```python
from build123d import *

# Parameters (mm, degrees)
F1_DEPTH = 10
F0_R     = 9.5
F2_DEPTH = 20
F3_DEPTH = 5
F4_R     = 6


with BuildPart() as f1:
    # F0 (on Top) → F1 (new body)
    with BuildSketch(Plane.XY):
        with BuildLine():
            Line((-9, 60), (-9, 42.0475920833))
            ThreePointArc((-9, 42.0475920833), (-6.5112727326, 42.5041565897), (-4, 42.8135492572))
            Line((-4, 42.8135492572), (-4, 60))
            ThreePointArc((-4, 60), (0, 64), (4, 60))
            Line((4, 60), (4, 42.8135492572))
            ThreePointArc((4, 42.8135492572), (6.5112727326, 42.5041565897), (9, 42.0475920833))
            Line((9, 42.0475920833), (9, 60))
            ThreePointArc((9, 60), (0, 69), (-9, 60))
        make_face()
        with BuildLine():
            Line((-9, 42.0475920833), (-9, 14.4222051019))
            ThreePointArc((-9, 14.4222051019), (0, 17), (9, 14.4222051019))
            Line((9, 14.4222051019), (9, 42.0475920833))
            ThreePointArc((9, 42.0475920833), (6.5112727326, 42.5041565897), (4, 42.8135492572))
            Line((4, 42.8135492572), (4, 33))
            ThreePointArc((4, 33), (0, 29), (-4, 33))
            Line((-4, 33), (-4, 42.8135492572))
            ThreePointArc((-4, 42.8135492572), (-6.5112727326, 42.5041565897), (-9, 42.0475920833))
        make_face()
    extrude(amount=F1_DEPTH)

    # F0 (on Top) → F2 (join)
    with BuildSketch(Plane.XY):
        with BuildLine():
            ThreePointArc((-9, 14.4222051019), (-8.2462112512, -14.8660687473), (17, 0))
            ThreePointArc((17, 0), (16.9906697283, 0.5631537833), (16.9626891549, 1.1256894045))
            ThreePointArc((16.9626891549, 1.1256894045), (14.5847399518, 8.7341491022), (9, 14.4222051019))
            ThreePointArc((9, 14.4222051019), (0, 17), (-9, 14.4222051019))
        make_face()
        Circle(F0_R, mode=Mode.SUBTRACT)
    extrude(amount=F2_DEPTH)

    # F0 (on Top) → F3 (join)
    with BuildSketch(Plane.XY):
        with BuildLine():
            ThreePointArc((9, 14.4222051019), (14.5847399518, 8.7341491022), (16.9626891549, 1.1256894045))
            ThreePointArc((16.9626891549, 1.1256894045), (19.3722847508, 6.3399805993), (25.0605147601, 7.1393697171))
            ThreePointArc((25.0605147601, 7.1393697171), (36.2055537239, 10.0321400586), (37.2390923627, 21.5))
            ThreePointArc((37.2390923627, 21.5), (25.2994921043, 34.7697526489), (9, 42.0475920833))
            Line((9, 42.0475920833), (9, 14.4222051019))
        make_face()
        with BuildLine():
            ThreePointArc((32.04293994, 18.5), (30.5788383249, 13.0358983849), (25.1147367097, 14.5))
            ThreePointArc((25.1147367097, 14.5), (20.5060966544, 20.5060966544), (14.5, 25.1147367097))
            ThreePointArc((14.5, 25.1147367097), (13.0358983849, 30.5788383249), (18.5, 32.04293994))
            ThreePointArc((18.5, 32.04293994), (26.1629509039, 26.1629509039), (32.04293994, 18.5))
        make_face(mode=Mode.SUBTRACT)
    extrude(amount=F3_DEPTH)

    # F4
    f4_edges = [f1.edges().sort_by_distance(p)[0] for p in [
        (9, 42.047592, 2.5),
    ]]
    fillet(f4_edges, radius=F4_R)


solid = f1.part
```
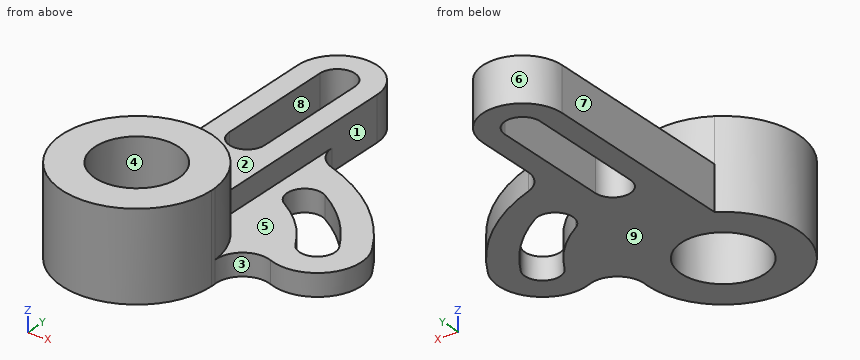
Check sheet for the modelled part. Datum: model origin and axes. Units: mm. Face numbers are marked on the shaded views. A direction names the side the tool comes from. Round coordinates to 2 decimals unless told otherwise and drop trailing zeros. Loops run counter-clockwise (first coordinate to the right, second up) from the corner with the lowest first, then second, coordinate; pieces in that order, holes last. Notation, with made-up numbers: (-31, 48.25) -> (-5, 48.25) arc R24 cw to (-5, 72.25) -> close; hole circle Ø11 at (-5.5, -12). An arc over 180 degrees is marked (long way). Answer in a Markdown table with one row per item.
Q1. Sectioned sample at A-A on y = 54. Enter the section's corners in (x, z).
Data:
| item | result |
|---|---|
| outline | (-9, 0) -> (-4, 0) -> (-4, 10) -> (-9, 10) -> close; (4, 0) -> (9, 0) -> (9, 10) -> (4, 10) -> close |
Q2. Go/stop test with flat-tipped pins: P1, Ø5, axis at y = 52.5, z = 5.5, coming from the -X side; P2, Ø14.5, axis at x = -1, y = 53, coming from the +Z side; P3, Ø11, axis at y = 36.5, z = 5, coming from the +X side; P4, Ø8, axis at y = 44, z = 16, coming from the -X side. Record where each tip stops, or that it passes through.
Data:
| item | result |
|---|---|
| P1 | stops at x = -9 |
| P2 | stops at z = 10 |
| P3 | stops at x = 29.8 |
| P4 | passes through |
Q3. Set-up check for the marked faces 5, 6, 7, 8 and 9: record each of +Z, -Z, +X, -X, +Y, -Y from which the full face is reachable in a straight line by a thin tool's end or side.
Data:
| item | result |
|---|---|
| face 5 | +Z, +X, +Y |
| face 6 | +Z, -Z, +Y |
| face 7 | +Z, -Z, -X, +Y |
| face 8 | +Z, -Z |
| face 9 | -Z, +X, -X, +Y, -Y |
Q4. Sectioned sample at D-D on y = 44. Enter the section's corners in (x, z).
Data:
| item | result |
|---|---|
| outline | (-9, 0) -> (-4, 0) -> (-4, 10) -> (-9, 10) -> close; (4, 0) -> (9.62, 0) -> (9.62, 5) -> (9, 5) -> (9, 10) -> (4, 10) -> close |
Q5. Sectioned sample at B-B on x = 5. Enter the section's corners in (y, z).
Data:
| item | result |
|---|---|
| outline | (-16.25, 0) -> (-8.08, 0) -> (-8.08, 20) -> (-16.25, 20) -> close; (8.08, 0) -> (67.48, 0) -> (67.48, 10) -> (16.25, 10) -> (16.25, 20) -> (8.08, 20) -> close |
Q6. Thickness scan on L1, parallel to X at y = 56, z = 1.25; L2, parallel to Y at x = 0, z = 15.75; L3, parallel to X at y = 27.5, z = 1. Record the ranges inside material, lowest first.
Data:
| item | result |
|---|---|
| L1 | x = -9 to -4, 4 to 9 |
| L2 | y = -17 to -9.5, 9.5 to 17 |
| L3 | x = -9 to 12.65, 24.75 to 33.06 |
Q7. Sectioned sample at C-C on z = 11.5. Enter the section's corners in (x, y).
Data:
| item | result |
|---|---|
| outline | circle Ø34 at (0, 0); hole circle Ø19 at (0, 0) |
Q8. Release check for a two-part mould opening along X. For the marked faces 1, 2, 3 and 4 record: released by +X, released by -X, zero draft, split by the parting line, or undercut.
Data:
| item | result |
|---|---|
| face 1 | released by +X |
| face 2 | zero draft |
| face 3 | undercut |
| face 4 | undercut |
